Could you check a few things on this model? Use its own coordinates, in mm. Face numbers are marked on the shaded views. A direction names the side the tool comes from. Give positions to 0.01 mm unless a question says otherwise; leave off trailing zeros. Write each loop counter-clockwise with the first axis right and the second up, starting at its lowest first coordinate (ties: lowest second). Pieces come first, ordered by that corner, then holes. Notation, with made-up numbers: (-12, 83.25) - (-7, 83.25) arc R12 ccw to (-7, 90.25) - close; hole circle Ø8 at (-32, 19). An arc over 180 degrees is marked (long way). Answer in a Markdown table with one row per item.
Autodesk Inventor part; units mm, degrees
ref_plane "YZ Plane" through (0, 0, 0) normal (1, 0, 0) x (0, 1, 0)
ref_plane "XZ Plane" through (0, 0, 0) normal (0, 1, 0) x (-1, 0, 0)
ref_plane "XY Plane" through (0, 0, 0) normal (0, 0, 1) x (1, 0, 0)
sketch "Sketch1" plane through (0, 0, 0) normal (0, 1, 0) x (-1, 0, 0)
  circle A0 centre (0, 0) radius 2.0828
  dimension "d4" = 4.1656
extrude "Body" add sketch "Sketch1" along normal blind 31.75
sketch "Sketch2" plane through (0, 0, 0) normal (1, 0, 0) x (0, 1, 0)
  line L0 (31.75, -2.0828) -> (31.75, 2.0828)
  line L1 (31.75, 0) -> (31.75, -3.9624)
  line L2 (31.75, -3.9624) -> (32.131, -3.9624)
  arc A0 (32.131, -3.9624) -> (33.9598, -2.0828) centre (29.9388, 0) ccw
  line L3 (33.9598, -2.0828) -> (33.9598, -1.6764)
  line L4 (33.9598, -1.6764) -> (32.4635, -1.6764)
  line L5 (32.4635, -1.6764) -> (31.8516, 0)
  line L6 (31.8516, 0) -> (31.75, 0)
  point P0 (0, 0)
  dimension "d5" = 3.9624
  dimension "d6" = 0.381
  dimension "d13" = 0.1016
  dimension "d14" = 2.0828
  dimension "d15" = 2.2098
  dimension "d16" = 0
  dimension "d17" = 1.6764
  dimension "d57" = 20.053
revolve "Head" add sketch "Sketch2" angle 360 about axis through (0, 31.8516, 0) along (0, -1, 0)
sketch "Sketch3" plane through (0, 33.9598, 0) normal (0, 1, 0) x (1, 0, 0)
  circle A0 centre (0, 0) radius 1.6764
  line L0 (0.7302, -1.2648) -> (-0.7303, -1.2648) construction
  line L1 (-0.7303, -1.2648) -> (-1.4605, 0) construction
  line L2 (-1.4605, 0) -> (-0.7303, 1.2648) construction
  line L3 (-0.7303, 1.2648) -> (0.7302, 1.2648) construction
  line L4 (0.7302, 1.2648) -> (1.4605, 0) construction
  line L5 (1.4605, 0) -> (0.7302, -1.2648) construction
  circle A1 centre (-0.7303, -1.2648) radius 0.2159
  circle A2 centre (-1.4605, 0) radius 0.2159
  circle A3 centre (-0.7303, 1.2648) radius 0.2159
  circle A4 centre (0.7302, 1.2648) radius 0.2159
  circle A5 centre (1.4605, 0) radius 0.2159
  circle A6 centre (0.7302, -1.2648) radius 0.2159
  circle A7 centre (0, -2.0701) radius 0.8712
  circle A8 centre (0, 2.0701) radius 0.8712
  circle A9 centre (1.7928, -1.0351) radius 0.8712
  circle A10 centre (-1.7928, 1.035) radius 0.8712
  circle A11 centre (1.7928, 1.035) radius 0.8712
  circle A12 centre (-1.7928, -1.0351) radius 0.8712
  circle A13 centre (0, 0) radius 1.8188
  point P0 (0, 0)
  point P1 (0, 0)
  point P2 (0.9413, 1.2192)
  point P3 (1.5265, 0.2056)
  point P4 (1.5265, -0.2056)
  point P5 (0.9413, -1.2192)
  point P6 (0.5852, -1.4248)
  point P7 (-0.5852, -1.4248)
  point P8 (-0.9413, -1.2192)
  point P9 (-1.5265, -0.2056)
  point P10 (-1.5265, 0.2056)
  point P11 (-0.9413, 1.2192)
  point P12 (-0.5852, 1.4248)
  point P13 (0.5852, 1.4248)
  dimension "d58" = 2.921
  dimension "d59" = 4.1402
  dimension "d62" = 120
extrude "Hex" add sketch "Sketch3" against normal blind 1.778 contours A5 A11 A0 | A0 A11 A13 A9 | A0 A9 A5 | A11 A0 | A0 A11 A13 | A9 A13 A0 | A0 A9 | A11 A4 A0 | A0 A8 A13 A11 | A9 A13 A7 A0 | A0 A6 A9 | A4 A8 A0 | A0 A7 A6 | A8 A0 | A7 A0 | A0 A8 A13 | A7 A13 A0 | A3 A0 A8 | A7 A0 A1 | A0 A10 A13 A8 | A7 A13 A12 A0 | A3 A10 A0 | A0 A12 A1 | A10 A0 A13 | A13 A12 A0 | A10 A0 | A0 A12 | A10 A0 A12 A13 | A10 A2 A0 | A0 A2 A12
sketch "Sketch4" plane through (0, 0, 0) normal (0, 0, 1) x (1, 0, 0)
  line L0 (-0.7364, 33.0198) -> (-1.6764, 33.9598)
  line L1 (0, 33.9598) -> (-0.7364, 33.0198)
  line L2 (0, -9.332) -> (0, 55.9918)
  line L3 (-1.5265, 33.9598) -> (-1.5265, 32.4138)
  line L4 (-1.5265, 33.9598) -> (-1.5265, 33.9598)
  line L5 (-1.5265, 33.9598) -> (-1.5265, 32.4138)
  line L6 (-1.6764, 33.9598) -> (-1.5265, 33.9598)
  line L7 (-1.6764, 33.9598) -> (0, 33.9598)
  point P0 (0, 0)
  point P1 (-1.6764, 32.4635)
  dimension "d29" = 1.6764
revolve "Head Chamfer" cut sketch "Sketch4" angle 360 about axis through (0, -10, 0) along (0, 1, 0)
feature "Thread" [suppressed]
sketch "Sketch6" plane through (0, 0, 0) normal (0, 0, 1) x (1, 0, 0)
  line L0 (0, 0) -> (-1.4859, 0)
  line L1 (2.0828, 0) -> (-2.0828, 0)
  line L2 (-1.4859, 0) -> (-2.4948, 1.0089)
  line L3 (-2.4948, 1.0089) -> (-2.9651, -1.2188)
  line L4 (-2.9651, -1.2188) -> (-1.4859, -1.2188)
  line L5 (-2.0828, 0) -> (-2.0828, 31.75)
  line L6 (-1.4859, -1.2188) -> (-1.4859, 0)
  line L7 (0, -10.3526) -> (0, 53.5838)
  point P0 (-2.0828, 0.5969)
  dimension "d49" = 1.4859
  dimension "d50" = 135
revolve "Tapered End" cut sketch "Sketch6" angle 360 about axis through (0, -10, 0) along (0, 1, 0)
sketch "Sketch8" plane through (0, 33.9598, 0) normal (0, 1, 0) x (1, 0, 0)
  circle A0 centre (0, 0) radius 4.7625
  point P0 (0, 0)
extrude "Extrusion3" cut sketch "Sketch8" against normal blind 1.016
sketch "Sketch5" plane through (0, 0, 0) normal (1, 0, 0) x (0, 1, 0)
  line L0 (0, -2.0828) -> (31.75, -2.0828)
  line L1 (31.75, 3.9624) -> (31.75, -3.9624)
  line L2 (31.75, -2.0828) -> (31.75, 2.0828)
  line L3 (0.0745, -2.0828) -> (-0.2261, -2.6035)
  line L4 (-0.2261, -2.6035) -> (-0.3253, -2.6035)
  line L5 (-0.3253, -2.6035) -> (-0.626, -2.0828)
  line L6 (0.0686, -2.6035) -> (-0.7252, -2.6035) construction
  line L7 (-0.626, -2.0828) -> (0.0745, -2.0828)
  line L8 (0, -2.0828) -> (31.75, -2.0828)
  point P0 (0, 0)
  dimension "d31" = 30
  dimension "d32" = 60
  dimension "a" = 0.0992
  dimension "d46" = 0.7937
  dimension "d54" = 0.0686
  dimension "d55" = 0.5207
  dimension "d56" = 0.0992
equation "\"d56\" = a"
properties part number "Screw 8-32 Steel 2.500" material "VEX Steel"
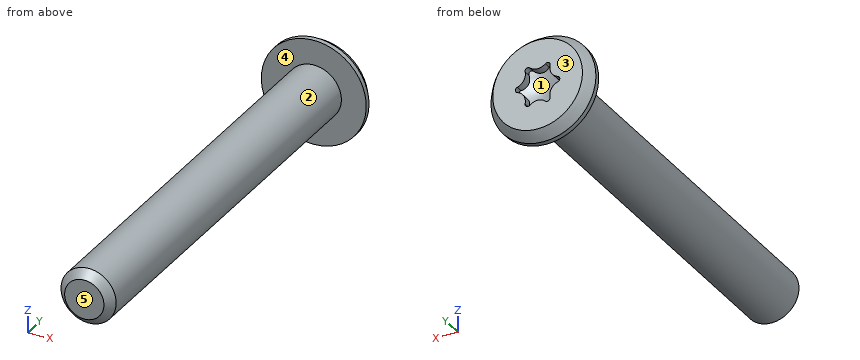
1) On a 3-axis mill with a long thin cutter (end or side, diameter ignored), from which of +Z, -Z, +X, -X, +Y, -Y can I reach the whole of each face in a straight line? I mean the marked faces 4 and 5. Say none if no direction works.
Check values:
| item | result |
|---|---|
| face 4 | -Y |
| face 5 | +Z, -Z, +X, -X, -Y |
2) If I drill on line 1 (Y direction, x = -2.25, z = -0.25); line 2 (X direction, y = 2.5, z = 0.25); line 3 (Y direction, x = 0.25, z = 3.5), over which ranges is the centre line in solid material (lowest first)?
Check values:
| item | result |
|---|---|
| line 1 | y = 31.75 to 32.94 |
| line 2 | x = -2.07 to 2.07 |
| line 3 | y = 31.75 to 32.8 |
3) Imagine slicing it at A-A (y = 14.5). List the corners of the cut face in (x, z) for me.
Check values:
| item | result |
|---|---|
| outline | circle Ø4.17 at (0, 0) |
4) We'd pull the mould along Z, two halves only. Please class the marked faces 1, 2 and 3: +Z half, -Z half, draft (parallel to the pull), parting line (faces both ways), or undercut.
Check values:
| item | result |
|---|---|
| face 1 | undercut |
| face 2 | parting line |
| face 3 | draft |
5) Will this pin go through, and if not, where does the flat tip stop? P1, Ø1, axis at x = 1.5, z = 2, coming from the -Y side.
Check values:
| item | result |
|---|---|
| P1 | stops at y = 0.51 |
